Source: CAD feature listing. Evaluate the final solid. Frame: model axes, mm. A direction names the side the tool comes from. Round coordinates to 2 decimals unless told otherwise and drop trailing zeros. Write each loop counter-clockwise with the first axis right and the second up, starting at its lowest first coordinate (ties: lowest second). Pieces come first, ordered by that corner, then holes. Notation, with made-up numbers: M -7,77.5 L -2,77.5 A31 ccw -2,115.5 Z; hole C 66.25,76.25 d11. An arc over 180 degrees is marked long. Answer in a Markdown table with one row per item. Add a question column.
Item 1: Cut plane B-B on z = 24.5. Return loops of the section in (x, y).
Item 2: Set-up query: faces 1 (the face through (-221.38, 3.13, 133.62)), 2 (the face through (-43, -12.7, 121)), 3 (the face through (216.613, 0, 69)). Return all of +Z, -Z, +X, -X, +Y, -Y with unobstructed straight access to the full face (end or side cutting, diameter ignored); none if empty.
Item 3: Contact query for flat-ended pins moving along their axis: pin 1 (1 mm diameter, centred on x = 44, y = 7, fed in from -Z); pin 2 (6 mm diameter, centred on x = -28.5, y = 6, fed in from +Z); pin 3 (13 mm diameter, centred on x = 0, z = 0, fed in from -Y); pin 4 (1 mm diameter, centred on x = 70, z = 132.5, fed in from -Y). Output: stop coordinate, or through.
Item 4: Mould query, pull axis Z, two halves, no side actions, for faces 4 (the face through (10, 0, 120.404)), 5 (the face through (-43, 12.7, 19)). Classes: released by +Z, released by -Z, zero draft, split by the parting line, or undercut.
Item 5: Material intervals for probe 1 along Z at (x, y) = (-120.5, 9.25); probe 2 along X at (y, z) = (-7.25, 70); probe 3 along X at (y, z) = (8, 7.5), sorted ascending.
Item 6: Cut plane C-C on z = 0. Return loops of the section in (x, y).
Item 7: Cut plane A-A on x = -82. Return loops of the section in (y, z), and give its area (3 significant figures).
from build123d import *

# Parameters (mm, degrees)
F4_D     = 11.1125
F4_DEPTH = 12.7011486273


# Not quite as in the source:
# - a length typed as a fraction of an inch, garbled in the dataset ("3 / 203.2 mm" for 3/8 in), is restored


with BuildPart() as f2:
    # F2: sweep along a path in F1
    with BuildLine(Plane.XZ) as f2_path:
        Line((235.9086840398, 0), (0, 0))
        Line((0, 0), (-221.2913159602, 0))
        Line((-221.2913159602, 0), (-221.2913159602, 139.7))
        Line((-221.2913159602, 139.7), (235.9086840398, 139.7))
        Line((235.9086840398, 139.7), (235.9086840398, 0))
    # F0 (on Right) → F2 (sweep)
    with BuildSketch(Plane.YZ):
        Polygon((-6.35, 7.5911765571), (-6.35, -7.5911765571), (-12.7001486273, -7.648065583), (-12.6998513727, -19.7300187742), (12.7001486273, -19.7165756275), (12.6998513727, -7.6346224362), (6.35, -7.5911765571), (6.35, 7.5911765571), (12.7, 7.5911765571), (12.7, 19.2955805858), (-12.7, 19.2955805858), (-12.7, 7.5911765571), align=None)
    sweep(path=f2_path.line, transition=Transition.RIGHT)

    # F4 (through all, one way)
    with BuildSketch(Plane.XZ):
        with Locations((-220.1733291149, 139.0449106693), (-220.1733291149, 0), (0, 139.0449106693), (0, 0), (234.9551618099, 139.0449106693), (234.9551618099, 0)):
            Circle(F4_D / 2)
    extrude(amount=-F4_DEPTH, mode=Mode.SUBTRACT)


solid = f2.part
Results below:
| question | item | result |
|---|---|---|
| 1 | outline | M -241.02,-12.7 L -228.94,-12.7 L -228.88,-6.35 L -213.7,-6.35 L -213.7,-12.7 L -202,-12.7 L -202,12.7 L -213.7,12.7 L -213.7,6.35 L -228.88,6.35 L -228.93,12.7 L -241.01,12.7 Z; M 216.61,-12.7 L 228.32,-12.7 L 228.32,-6.35 L 243.5,-6.35 L 243.56,-12.7 L 255.64,-12.7 L 255.63,12.7 L 243.54,12.7 L 243.5,6.35 L 228.32,6.35 L 228.32,12.7 L 216.61,12.7 Z |
| 2 | face 1 | +Y |
| 2 | face 2 | +Z, -Z, +X, -X, -Y |
| 2 | face 3 | +Y, -Y |
| 3 | pin 1 | z = -19.72 |
| 3 | pin 2 | z = 159.42 |
| 3 | pin 3 | y = -6.35 |
| 3 | pin 4 | y = -12.7 |
| 4 | face 4 | undercut |
| 4 | face 5 | zero draft |
| 5 | probe 1 | -19.72 to -7.61, 7.59 to 19.3, 120.4 to 132.11, 147.31 to 159.42 |
| 5 | probe 2 | -241.02 to -228.89, -213.7 to -202, 216.61 to 228.32, 243.51 to 255.64 |
| 5 | probe 3 | -241.01 to -228.89, 243.51 to 255.63 |
| 6 | outline | M -241.02,-12.7 L -228.94,-12.7 L -228.88,-6.35 L 243.5,-6.35 L 243.56,-12.7 L 255.64,-12.7 L 255.63,12.7 L 243.54,12.7 L 243.5,6.35 L 240.51,6.35 L 240.51,0 L 229.4,0 L 229.4,6.35 L 5.56,6.35 L 5.56,0 L -5.56,0 L -5.56,6.35 L -214.62,6.35 L -214.62,0 L -225.73,0 L -225.73,6.35 L -228.88,6.35 L -228.93,12.7 L -241.01,12.7 Z |
| 7 | outline | M -12.7,-19.73 L 12.7,-19.72 L 12.7,-7.63 L 6.35,-7.59 L 6.35,7.59 L 12.7,7.59 L 12.7,19.3 L -12.7,19.3 L -12.7,7.59 L -6.35,7.59 L -6.35,-7.59 L -12.7,-7.65 Z; M -12.7,120.4 L 12.7,120.4 L 12.7,132.11 L 6.35,132.11 L 6.35,147.29 L 12.7,147.33 L 12.7,159.42 L -12.7,159.43 L -12.7,147.35 L -6.35,147.29 L -6.35,132.11 L -12.7,132.11 Z |
| 7 | area | 1,600 mm2 |
